Answer from the drawing. Dimensions are ordinates in mm from the lowest x, y and z of the part. A direction names the side the tool comes from. Round coordinates to 2 decimals unless told otherwise and drop trailing zeros. Loops run counter-clockwise (first coordinate to the right, second up) from the corner with the lowest first, then second, coordinate; pieces in that order, holes last.
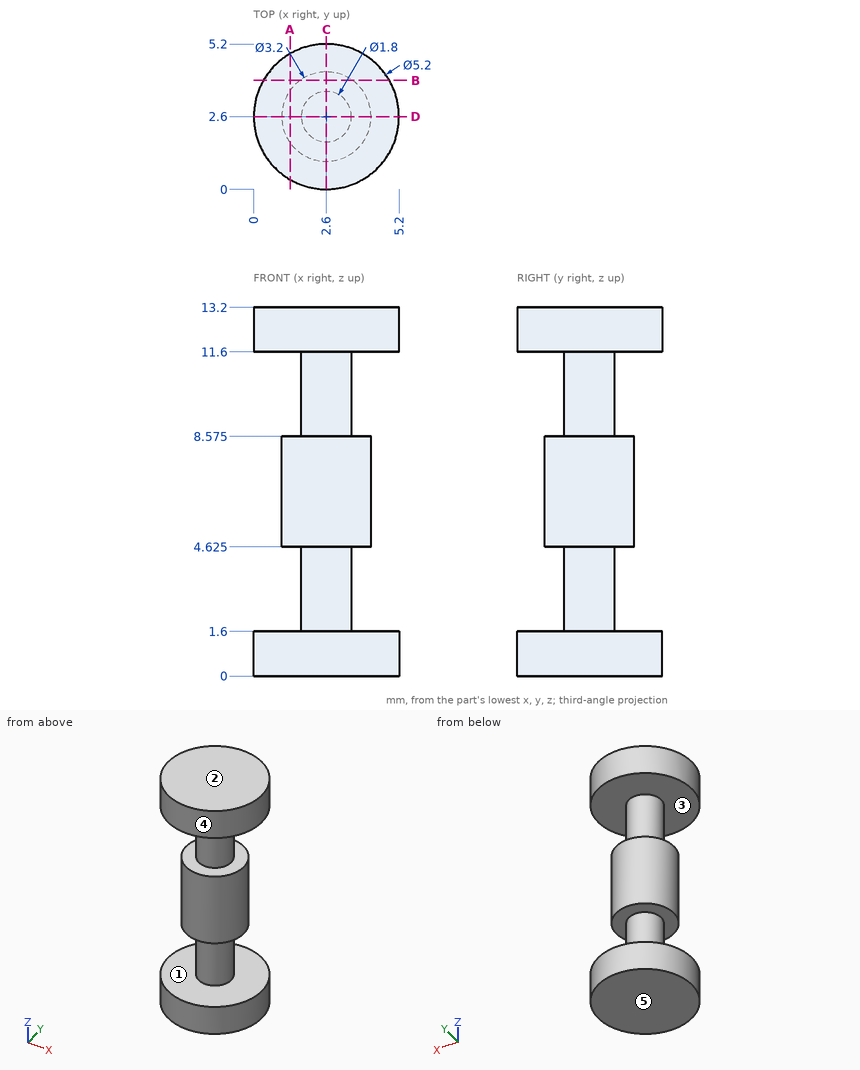
Item 1: Section C-C, the plane x = 2.6 is taken. Give the vertices of the cut face in (y, z) (3 decimals), plus the area to 3 significant figures.
Item 2: Section A-A, the plane x = 1.3 is taken. Give the vertices of the cut face in (y, z) (3 decimals), plus the area to 3 significant figures.
Item 3: Each of these flat-tipped pins is pushed along its axis until it touches: P1, Ø2, axis at y = 2, z = 7, coming from the +X side; P2, Ø1, axis at x = 2.5, y = 3, coming from the -Z side. Where does it stop, or does it pass through?
Item 4: For the marked faces 1 and 2, determine the directions among +Z, -Z, +X, -X, +Y, -Y from which every point of the face is accessible in a straight line to the end or side of a thin tool.
Item 5: Straight lines are drawn through the part: line 1 (Z direction, x = 3.4, y = 1.35) (3 decimals); line 2 (Z direction, x = 1.65, y = 0.3); line 3 (X direction, y = 2.55, z = 4.5). For each, find the intervals that lie inside material, in ascending order.
Item 6: Determine the mould class of the marked faces 3, 4 and 5 for opening direction Z: pulls with the +Z half, pulls with the -Z half, needs draft (parallel to the pull), parting line crosses it, or undercut.
Answer below:
1. outline: (0, 0) - (5.2, 0) - (5.2, 1.6) - (3.5, 1.6) - (3.5, 4.625) - (4.2, 4.625) - (4.2, 8.575) - (3.5, 8.575) - (3.5, 11.6) - (5.2, 11.6) - (5.2, 13.2) - (0, 13.2) - (0, 11.6) - (1.7, 11.6) - (1.7, 8.575) - (1, 8.575) - (1, 4.625) - (1.7, 4.625) - (1.7, 1.6) - (0, 1.6) - close
1. area: 40.2 mm2
2. outline: (0.348, 0) - (4.852, 0) - (4.852, 1.6) - (0.348, 1.6) - close; (0.348, 11.6) - (4.852, 11.6) - (4.852, 13.2) - (0.348, 13.2) - close; (1.667, 4.625) - (3.533, 4.625) - (3.533, 8.575) - (1.667, 8.575) - close
2. area: 21.8 mm2
3. P1: stops at x = 4.2
3. P2: stops at z = 0
4. face 1: none
4. face 2: +Z, +X, -X, +Y, -Y
5. line 1: z = 0 to 1.6, 4.625 to 8.575, 11.6 to 13.2
5. line 2: z = 0 to 1.6, 11.6 to 13.2
5. line 3: x = 1.7 to 3.5
6. face 3: undercut
6. face 4: needs draft
6. face 5: pulls with the -Z half
